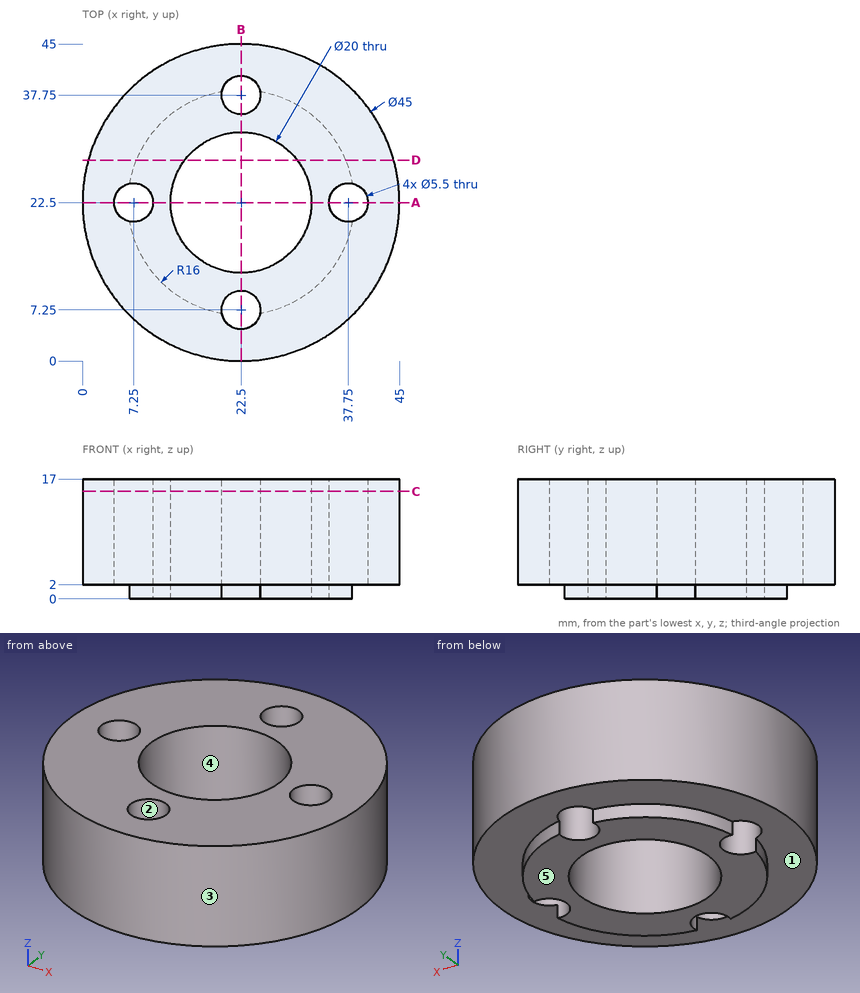
Here's the drawing with two shaded views (mm, measured from the low corner). I have some questions. A direction names the side the tool comes from. Give positions to 0.01 mm unless a question says otherwise; leave off trailing zeros. Loops run counter-clockwise (first coordinate to the right, second up) from the corner with the lowest first, then second, coordinate; pieces in that order, holes last. Notation, with made-up numbers: M 85,42.25 L 92,42.25 A20 ccw 92,50.25 Z; hole C 23.25,69.25 d11. An arc over 180 degrees is marked long. One line per item, written item: value. Start each with the question number.
1) Thinking about a two-plate mould opening in Y: for the marked faces 3, 4 and 5, which applies, +Y half, -Y half, draft (parallel to the pull), parting line (faces both ways), or undercut?
2) If we section it at A-A, the plane y = 22.5: Write out the boundary of the cut face in (x, z).
3) If we section it at C-C, the plane z = 15.25: Write out the boundary of the cut face in (x, y).
4) On a 3-axis mill with a long thin cutter (end or side, diameter ignored), from which of +Z, -Z, +X, -X, +Y, -Y can I reach the whole of each face in a straight line? I mean the marked faces 1 and 2. Say none if no direction works.
5) If we section it at D-D, the plane y = 28.5: Write out the boundary of the cut face in (x, z).
6) I'm going to push flat-ended pins straight in: pin 1 (5 mm diameter, centred on x = 22.5, y = 7.25, fed in from +Z); pin 2 (5 mm diameter, centred on x = 20.5, y = 37.5, fed in from +Z); pin 3 (4 mm diameter, centred on x = 13.5, z = 13.5, fed in from -Y); pin 4 (1.5 mm diameter, centred on y = 10, z = 5.5, fed in from +X). Where does each tip first touch, or does it pass through?
7) If I drill on line 1 (Y direction, x = 22.5, z = 8); line 2 (X direction, y = 23.5, z = 8.75); line 3 (Y direction, x = 37.75, z = 7.75), over which ranges is the centre line in solid material (lowest first)? Write a range as [from, to].
Completed:
1. face 3: parting line
1. face 4: undercut
1. face 5: draft
2. outline: M 0,2 L 4.5,2 L 4.5,17 L 0,17 Z; M 10,0 L 12.5,0 L 12.5,17 L 10,17 Z; M 32.5,0 L 35,0 L 35,17 L 32.5,17 Z; M 40.5,2 L 45,2 L 45,17 L 40.5,17 Z
3. outline: C 22.5,22.5 d45; hole C 7.25,22.5 d5.5; hole C 22.5,22.5 d20; hole C 22.5,7.25 d5.5; hole C 22.5,37.75 d5.5; hole C 37.75,22.5 d5.5
4. face 1: -Z
4. face 2: +Z, -Z
5. outline: M 0.81,2 L 7.67,2 L 7.67,0 L 14.5,0 L 14.5,17 L 0.81,17 Z; M 30.5,0 L 37.33,0 L 37.33,2 L 44.19,2 L 44.19,17 L 30.5,17 Z
6. pin 1: passes through
6. pin 2: stops at z = 17
6. pin 3: stops at y = 1.12
6. pin 4: stops at x = 41.69
7. line 1: y = [0, 4.5], [10, 12.5], [32.5, 35], [40.5, 45]
7. line 2: x = [0.02, 4.69], [9.81, 12.55], [32.45, 35.19], [40.31, 44.98]
7. line 3: y = [5.96, 19.75], [25.25, 39.04]
